The drawing under review shows one solid part. Ordinate dimensions are in mm from its lowest x, y, z. A direction names the side the tool comes from. Coordinates: 2 decimals unless noted, no trailing zeros. Order: outer loops, then holes, each group sorted by start corner. A loop starts at its lowest first (then second) coordinate and runs counter-clockwise, first axis right, second up. Notation, with made-up numbers: (-28.75, -9.5) -> (12.25, -9.5) arc R23 ccw to (12.25, 1.5) -> close; hole circle Ø11 at (38.25, 3.5). An arc over 180 degrees is marked (long way). Use a Markdown table: item, result. Add a question column.
Q1. Add section A-A (z = 7.5). State the section outline as (x, y) points.
Q2. The part is to be moulded in two halves that separate along Z. For the marked faces 4, 5, 6 and 7, say which applies: pulls with the +Z half, pulls with the -Z half, needs draft (parallel to the pull), parting line crosses it, or undercut.
Q3. Wall thickness on probe 1 along Y at (x, z) = (4.5, 10.5); probe 2 along X at (y, z) = (20.5, 7.5); probe 3 along Z at (x, y) = (12.75, 9.75): over which ranges is each line inside the solid? List them lowest first.
Q4. Add section D-D (z = 14). State the section outline as (x, y) points, then the cut area to 3 significant figures.
Q5. Add section C-C (x = 12.5). State the section outline as (y, z) points, then the cut area to 3 significant figures.
Q6. Add section B-B (y = 2). State the section outline as (x, z) points, then the cut area to 3 significant figures.
Q7. Machinability: for the marked faces 1, 2 and 3, which of the approach directions +Z, -Z, +X, -X, +Y, -Y give a long, thin tool a straight path to every point of the face, cutting with its end or side? Answer none if there is none.
Q8. Insertion check: pin 1 (8 mm diameter, centred on y = 9.5, z = 5.5, fed in from +X); pin 2 (6 mm diameter, centred on y = 15, z = 12.5, fed in from +X); pin 3 (2 mm diameter, centred on y = 17, z = 8, fed in from +X). Each pin has a flat end and moves straight along its axis. Give the tip position at first contact, or say it passes through.
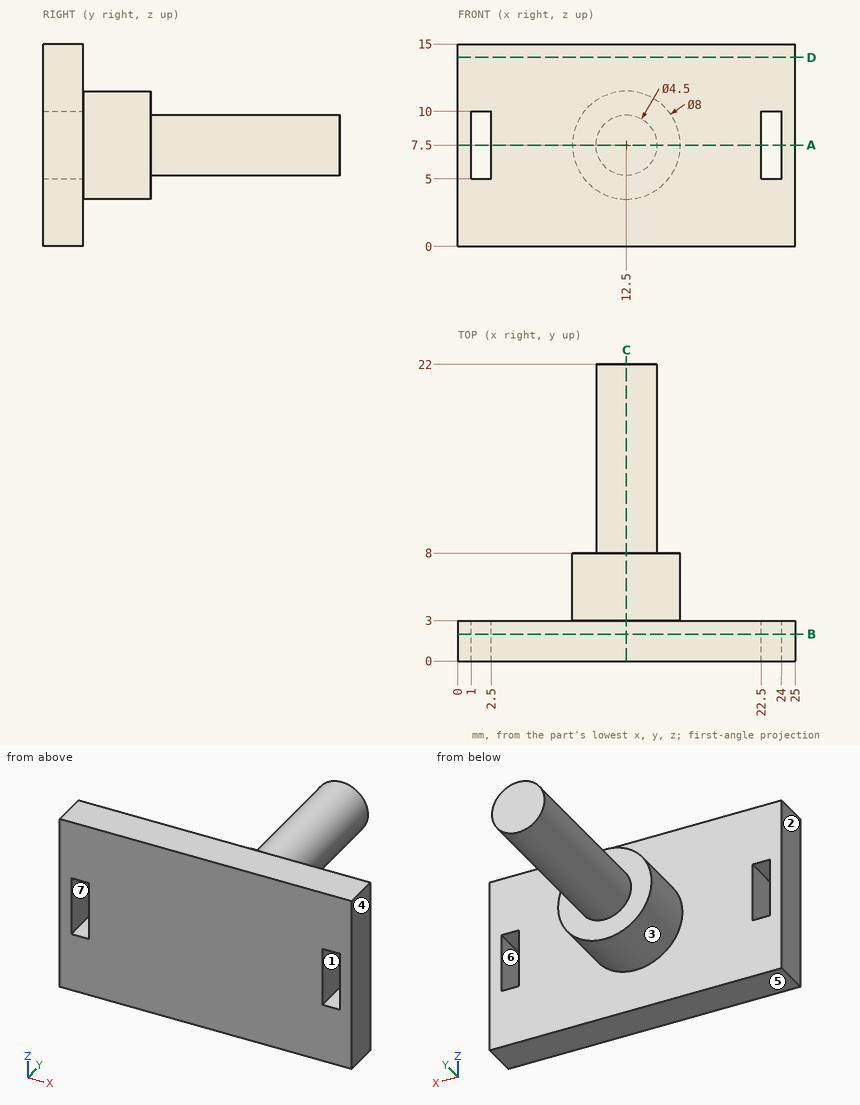
Established:
| question | item | result |
|---|---|---|
| 1 | outline | (0, 0) -> (1, 0) -> (1, 3) -> (0, 3) -> close; (2.5, 0) -> (22.5, 0) -> (22.5, 3) -> (16.5, 3) -> (16.5, 8) -> (14.75, 8) -> (14.75, 22) -> (10.25, 22) -> (10.25, 8) -> (8.5, 8) -> (8.5, 3) -> (2.5, 3) -> close; (24, 0) -> (25, 0) -> (25, 3) -> (24, 3) -> close |
| 2 | face 4 | needs draft |
| 2 | face 5 | pulls with the -Z half |
| 2 | face 6 | undercut |
| 2 | face 7 | undercut |
| 3 | probe 1 | 0 to 3 |
| 3 | probe 2 | 10.25 to 14.75 |
| 3 | probe 3 | 5.26 to 9.74 |
| 4 | outline | (0, 0) -> (25, 0) -> (25, 3) -> (0, 3) -> close |
| 4 | area | 75.0 mm^2 |
| 5 | outline | (0, 0) -> (3, 0) -> (3, 3.5) -> (8, 3.5) -> (8, 5.25) -> (22, 5.25) -> (22, 9.75) -> (8, 9.75) -> (8, 11.5) -> (3, 11.5) -> (3, 15) -> (0, 15) -> close |
| 5 | area | 148 mm^2 |
| 6 | outline | (0, 0) -> (25, 0) -> (25, 15) -> (0, 15) -> close; hole (1, 5) -> (2.5, 5) -> (2.5, 10) -> (1, 10) -> close; hole (22.5, 5) -> (24, 5) -> (24, 10) -> (22.5, 10) -> close |
| 6 | area | 360 mm^2 |
| 7 | face 1 | +Y, -Y |
| 7 | face 2 | +Z, -Z, -X, +Y, -Y |
| 7 | face 3 | +Y |
| 8 | pin 1 | x = 16.5 |
| 8 | pin 2 | x = 13.53 |
| 8 | pin 3 | x = 14.75 |
